Autodesk Inventor part; units mm, degrees
ref_plane "YZ Plane" through (0, 0, 0) normal (1, 0, 0) x (0, 1, 0)
ref_plane "XZ Plane" through (0, 0, 0) normal (0, 1, 0) x (-1, 0, 0)
ref_plane "XY Plane" through (0, 0, 0) normal (0, 0, 1) x (1, 0, 0)
sketch "Sketch1" plane through (0, 0, 0) normal (0, 0, 1) x (1, 0, 0)
  line L0 (0, 0) -> (2, 0)
  line L1 (2, 0) -> (2, 16)
  line L2 (2, 16) -> (0, 16)
  line L3 (0, 16) -> (0, 0)
  line L4 (2, 2) -> (8, 2)
  line L5 (8, 2) -> (8, 0)
  line L6 (8, 0) -> (2, 0)
  line L7 (2, 0) -> (2, 2)
  dimension "d0" = 2
  dimension "d1" = 16
  dimension "d2" = 6
extrude "Extrusion1" add sketch "Sketch1" against normal blind 22
sketch "Sketch3" plane through (2, 2, 0) normal (1, 0, 0) x (0, 0, -1)
  line L0 (9.5, 14) -> (4.5, 14)
  line L1 (4.5, 14) -> (4.5, 8)
  line L2 (4.5, 8) -> (9.5, 8)
  line L3 (9.5, 8) -> (9.5, 14)
  point P0 (0, -2)
  dimension "d9" = 5
  dimension "d10" = 6
extrude "Extrusion3" cut sketch "Sketch3" against normal blind 10
properties part number "housing_mate_v05"
Read the model definition and answer for the solid it produces. Units are mm, in the model's axes. A direction names the side the tool comes from. Coordinates: 2 decimals unless noted, no trailing zeros. Write each loop counter-clockwise with the first axis right and the second up, starting at its lowest first coordinate (ties: lowest second). Pieces come first, ordered by that corner, then holes. Notation, with made-up numbers: (65, 55.5) - (82, 55.5) arc R6 ccw to (82, 65.5) - close; hole circle Ø3 at (51, 47.5). An arc over 180 degrees is marked (long way). One line per question, with ' | ' between items.
Q1. Find section C-C, the plane x = 1.75. Write down the section's boundary in (y, z), plus the area to 3 significant figures.
Result set:
outline: (0, -22) - (16, -22) - (16, -9.5) - (10, -9.5) - (10, -4.5) - (16, -4.5) - (16, 0) - (0, 0) - close | area: 322 mm^2
Q2. Each of these flat-tipped pins is pushed along its axis until it touches: P1, Ø7, axis at y = 7, z = -8.5, coming from the +X side; P2, Ø1.8, axis at x = 4.5, z = -8.5, coming from the +Y side; P3, Ø0.6, axis at x = 0.5, z = -6.5, coming from the +Y side. Where does it stop, or does it pass through?
Result set:
P1: x = 2 | P2: y = 2 | P3: y = 10
Q3. Find section B-B, the plane z = -3. Write down the section's boundary in (x, y).
Result set:
outline: (0, 0) - (8, 0) - (8, 2) - (2, 2) - (2, 16) - (0, 16) - close
Q4. Find section A-A, the plane y = 11. Write down the section's boundary in (x, z).
Result set:
outline: (0, -22) - (2, -22) - (2, -9.5) - (0, -9.5) - close; (0, -4.5) - (2, -4.5) - (2, 0) - (0, 0) - close
Q5. Determine the mould class of faces 4 (the flat face through (1, 10, -7)), 5 (the flat face through (1.6, 5.7, 0)), 6 (the flat face through (1.6, 5.7, -22)), 7 (the flat face through (5, 2, -11)) for opening direction Z: +Z half, -Z half, draft (parallel to the pull), parting line (faces both ways), or undercut.
Result set:
face 4: undercut | face 5: +Z half | face 6: -Z half | face 7: draft
Q6. Consider L1, parallel to X at y = 3.5, z = -15.5; L2, parallel to Z at x = 1, y = 11.5. Determine where each line is inside the solid, lowest interval first. Write a range as [from, to].
Result set:
L1: [0, 2] | L2: [-22, -9.5], [-4.5, 0]
Q7. Find section D-D, the plane y = 3.75. Write down the section's boundary in (x, z), plus the area to 3 significant figures.
Result set:
outline: (0, -22) - (2, -22) - (2, 0) - (0, 0) - close | area: 44.0 mm^2
Q8. For faces 1 (the flat face through (1, 13, -4.5)), 2 (the flat face through (2, 9, -11)), 3 (the flat face through (1, 16, -2)), determine the directions among +Z, -Z, +X, -X, +Y, -Y from which every point of the face is accessible in a straight line to the end or side of a thin tool.
Result set:
face 1: +X, -X, +Y | face 2: +Z, -Z, +X, +Y | face 3: +Z, -Z, +X, -X, +Y
